```python
from build123d import *

# Parameters (mm, degrees)
F0_W     = 110.998
F0_H     = 40.64
F1_DEPTH = 44.196
F5_D     = 22.098
F2_R     = 6.985
F6_DEPTH = 44.197
F7_DEPTH = 44.197
F3_W     = 64.77
F3_H     = 14.732
F8_DEPTH = 40.641
F9_DEPTH = 40.641


with BuildPart() as f1:
    # F0 (on Top) → F1 (new body)
    with BuildSketch(Plane.XY):
        with Locations((55.499, 20.32)):
            Rectangle(F0_W, F0_H)
    extrude(amount=F1_DEPTH)

    # F5 (through all)
    with Locations(Plane.XZ):
        with Locations((22.098, 22.098)):
            Hole(F5_D / 2)

    # F2 (on face) → F6 (cut, through all)
    with BuildSketch(Plane.XY.offset(44.196)):
        with Locations((90.678, 20.32)):
            Circle(F2_R)
    extrude(amount=-F6_DEPTH, mode=Mode.SUBTRACT)

    # F2 (on face) → F7 (cut, through all)
    with BuildSketch(Plane.XY.offset(44.196)):
        with BuildLine():
            ThreePointArc((90.678, 40.64), (105.0464097937, 34.6884097937), (110.998, 20.32))
            Line((110.998, 20.32), (110.998, 40.64))
            Line((110.998, 40.64), (90.678, 40.64))
        make_face()
        with BuildLine():
            Line((110.998, 0), (110.998, 20.32))
            ThreePointArc((110.998, 20.32), (105.0464097937, 5.9515902063), (90.678, 0))
            Line((90.678, 0), (110.998, 0))
        make_face()
    extrude(amount=-F7_DEPTH, mode=Mode.SUBTRACT)

    # F3 (on face) → F8 (cut, through all)
    with BuildSketch(Plane.XZ):
        with Locations((78.613, 22.098)):
            Rectangle(F3_W, F3_H)
    extrude(amount=-F8_DEPTH, mode=Mode.SUBTRACT)

    # F3 (on face) → F9 (cut, through all)
    with BuildSketch(Plane.XZ):
        with BuildLine():
            ThreePointArc((0, 22.098), (6.4723544116, 37.7236457129), (22.098000176, 44.196))
            Line((22.098000176, 44.196), (0, 44.196))
            Line((0, 44.196), (0, 22.098))
        make_face()
        with BuildLine():
            Line((0, 0), (22.098, 0))
            ThreePointArc((22.098, 0), (6.4723543493, 6.4723543493), (0, 22.098))
            Line((0, 22.098), (0, 0))
        make_face()
    extrude(amount=-F9_DEPTH, mode=Mode.SUBTRACT)


solid = f1.part
```
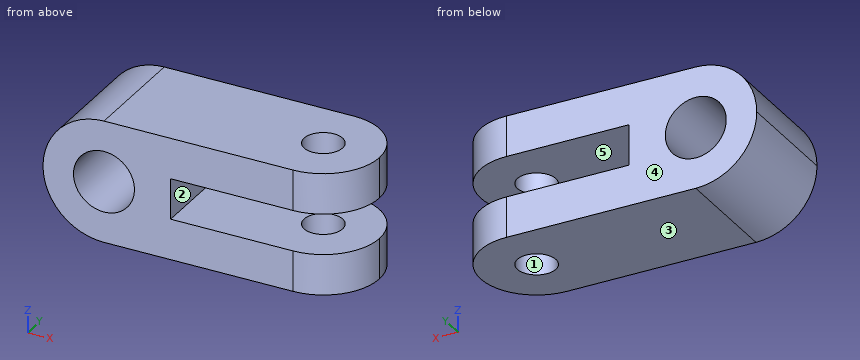
Source: CAD feature listing. Evaluate the final solid. Frame: model axes, mm. Face numbers are marked on the shaded views. A direction names the side the tool comes from. Coordinates: 2 decimals unless noted, no trailing zeros. Write each loop counter-clockwise with the first axis right and the second up, starting at its lowest first coordinate (ties: lowest second). Pieces come first, ordered by that corner, then holes. Notation, with made-up numbers: (81, 77) -> (93, 77) arc R21 ccw to (93, 92) -> close; hole circle Ø6 at (50, 79). An arc over 180 degrees is marked (long way). Return JSON: item names as keys, results as strings. Group by question number.
1) Mould query, pull axis X, two halves, no side actions, for the marked faces 1, 2 and 3. Classes: +X half, -X half, draft (parallel to the pull), parting line (faces both ways), or undercut.
2) Set-up query: the marked faces 4 and 5. Return all of +Z, -Z, +X, -X, +Y, -Y with unobstructed straight access to the full face (end or side cutting, diameter ignored); none if empty.
3) Section query D-D, the plane z = 8. Return loops of the section in (x, y) (3 decimals).
4) Section query A-A, the plane x = 70.5. Return loops of the section in (y, z), plus the area to 3 significant figures.
5) Section query B-B, the plane y = 25.5. Return loops of the section in (x, z).
6) Section query C-C, the plane y = 10. Return loops of the section in (x, z).
7) Ray query, line 1 along Z through (x, y) = (93.5, 3.5); line 2 along X through (y, z) = (25, 25); line 3 along X through (y, z) = (9, 32). Return the intervals inside material, ascending.
8) Contact query for flat-ended pins moving along their axis: P1, Ø3, axis at y = 32, z = 12.5, coming from the -X side; P2, Ø4.5, axis at y = 21, z = 22.5, coming from the +X side; P3, Ø1, axis at x = 19, y = 23.5, coming from the +Z side. Output: stop coordinate, or through.
From the geometry:
{
 "1": {"face 1": "undercut", "face 2": "+X half", "face 3": "draft"},
 "2": {"face 4": "+Z, -Z, +X, -X, +Y", "face 5": "+X, +Y, -Y"},
 "3": {"outline": "(5.081, 0) -> (90.678, 0) arc R20.32 ccw to (90.678, 40.64) -> (5.081, 40.64) -> close; hole circle Ø13.97 at (90.678, 20.32)"},
 "4": {"outline": "(0, 0) -> (40.64, 0) -> (40.64, 14.73) -> (0, 14.73) -> close; (0, 29.46) -> (40.64, 29.46) -> (40.64, 44.2) -> (0, 44.2) -> close", "area": "1,200 mm²"},
 "5": {"outline": "(22.1, 0) -> (85.99, 0) -> (85.99, 14.73) -> (46.23, 14.73) -> (46.23, 29.46) -> (85.99, 29.46) -> (85.99, 44.2) -> (22.1, 44.2) arc R22.1 ccw to start; (95.36, 0) -> (110.33, 0) -> (110.33, 14.73) -> (95.36, 14.73) -> close; (95.36, 29.46) -> (110.33, 29.46) -> (110.33, 44.2) -> (95.36, 44.2) -> close; hole circle Ø22.1 at (22.1, 22.1)"},
 "6": {"outline": "(22.1, 0) -> (108.18, 0) -> (108.18, 14.73) -> (46.23, 14.73) -> (46.23, 29.46) -> (108.18, 29.46) -> (108.18, 44.2) -> (22.1, 44.2) arc R22.1 ccw to start; hole circle Ø22.1 at (22.1, 22.1)"},
 "7": {"line 1": "0 to 14.73, 29.46 to 44.2", "line 2": "0.19 to 11.44, 32.76 to 46.23", "line 3": "2.34 to 17.2, 27 to 107.55"},
 "8": {"P1": "x = 1.54", "P2": "x = 46.23", "P3": "z = 44.04"}
}
